from build123d import *

# Parameters (mm, degrees)
SKETCH1_W           = 32
SKETCH1_H           = 24
BOSS_EXTRUDE1_DEPTH = 3
SKETCH2_R           = 3.5
BOSS_EXTRUDE2_DEPTH = 5
SKETCH3_W           = 5
SKETCH3_H           = 10
BOSS_EXTRUDE3_DEPTH = 3


with BuildPart() as part:
    # Sketch1 → Boss-Extrude1 (new body)
    with BuildSketch(Plane(origin=(0, 0, 0), x_dir=(1, 0, 0), z_dir=(0, 1, 0))):
        with Locations((0.62745098, -0.470588235)):
            Rectangle(SKETCH1_W, SKETCH1_H)
    extrude(amount=BOSS_EXTRUDE1_DEPTH)

    # Sketch2 → Boss-Extrude2 (add)
    with BuildSketch(Plane(origin=(0, 3, 0), x_dir=(1, 0, 0), z_dir=(0, 1, 0))):
        with Locations((1.078230838, 6.529411765)):
            Circle(SKETCH2_R)
        with Locations((9.078230838, 6.529411765)):
            Circle(SKETCH2_R)
    extrude(amount=BOSS_EXTRUDE2_DEPTH)

    # Sketch3 → Boss-Extrude3 (add)
    with BuildSketch(Plane(origin=(0, 3, 0), x_dir=(1, 0, 0), z_dir=(0, 1, 0))):
        with Locations((6.12745098, -3.470588235)):
            Rectangle(SKETCH3_W, SKETCH3_H)
    extrude(amount=BOSS_EXTRUDE3_DEPTH)


solid = part.part
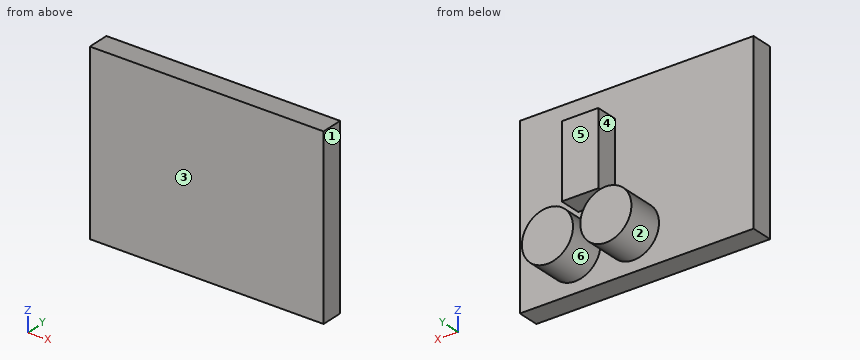
The listing builds one solid part. Answer for the finished solid, in the listing's coordinates (mm). Face numbers are marked on the shaded views. A direction names the side the tool comes from. Round coordinates to 2 decimals unless told otherwise and drop trailing zeros. Write each loop counter-clockwise with the first axis right and the second up, starting at its lowest first coordinate (ties: lowest second). Pieces come first, ordered by that corner, then holes. Notation, with made-up numbers: (56.25, 50) - (73.25, 50) arc R20 cw to (73.25, 86) - close; hole circle Ø11 at (41.25, 69.25). An arc over 180 degrees is marked (long way). Use one line per item in the form item = value. Start each with the question number.
Item 1: Find the intervals of material crossed by line 1 (X direction, y = 4, z = 1.5); line 2 (Y direction, x = 13.5, z = -5.5); line 3 (X direction, y = 6, z = -5), in increasing order. Write a range as [from, to].
Item 2: A cutting plane is placed at B-B (z = -0.5). Write down the section's boundary in (x, y).
Item 3: A cutting plane is placed at D-D (y = 3.75). Write down the section's boundary in (x, z), plus the area to 3 significant figures.
Item 4: Determine the mould class of the marked faces 1, 2 and 3 for opening direction X: +X half, -X half, draft (parallel to the pull), parting line (faces both ways), or undercut.
Item 5: A cutting plane is placed at C-C (y = 7.5). Write down the section's boundary in (x, z), plus the area to 3 significant figures.
Item 6: A tool of negligible diameter and unlimited length cuts with its end or side. For the marked faces 4, 5 and 6, from which of +Z, -Z, +X, -X, +Y, -Y can it reach the whole face along a straight path? Write none if from no direction.
Item 7: A cutting plane is placed at A-A (x = 11). Write down the section's boundary in (y, z).
Item 8: Flat-ended cylindrical pins translate along their axes: pin 1 Ø5.5 at (x, z) = (6.5, 1) entering from +Y; pin 2 Ø0.9 at (x, y) = (5.5, 4.5) entering from +Z; pin 3 Ø4 at (x, y) = (-3.5, 7) entering from +Z; pin 4 Ø5 at (x, z) = (-6, -3.5) entering from -Y. Find the tip coordinate at first contact, or state that the pin passes through.
The answers:
q1.line_1 = [3.63, 8.63]
q1.line_2 = [0, 3]
q1.line_3 = [-2.07, 4.23], [5.93, 12.23]
q2.outline = (-15.37, 0) - (16.63, 0) - (16.63, 3) - (8.63, 3) - (8.63, 6) - (3.63, 6) - (3.63, 3) - (-15.37, 3) - close
q3.outline = circle Ø7 at (1.08, -6.53); (3.63, -1.53) - (8.63, -1.53) - (8.63, 8.47) - (3.63, 8.47) - close; circle Ø7 at (9.08, -6.53)
q3.area = 127 mm^2
q4.face_1 = +X half
q4.face_2 = undercut
q4.face_3 = draft
q5.outline = circle Ø7 at (1.08, -6.53); circle Ø7 at (9.08, -6.53)
q5.area = 77.0 mm^2
q6.face_4 = +Z, -X, +Y
q6.face_5 = +Z, +X, -X, +Y
q6.face_6 = +Y
q7.outline = (0, -11.53) - (3, -11.53) - (3, -9.45) - (8, -9.45) - (8, -3.6) - (3, -3.6) - (3, 12.47) - (0, 12.47) - close
q8.pin_1 = 6
q8.pin_2 = 8.47
q8.pin_3 = -4.16
q8.pin_4 = 0
